from build123d import *

# Parameters (mm, degrees)
F1_DEPTH = 25.4
F3_R     = 39.2915838244
F4_DEPTH = 25.4
F6_R     = 62.7093604839
F7_DEPTH = 25.4
F8_T     = -2.54


with BuildPart() as f1:
    # F0 (on Front) → F1 (new body)
    with BuildSketch(Plane.XZ):
        with BuildLine():
            add(Edge.make_bspline(
                [(-55.208299309, 58.1508763134), (-67.0164708846, 55.3175541912), (-87.6445105915, -47.0922011076), (101.1268779134, 10.7779345683), (-19.4909088182, 79.2065756794), (-30.9714891326, 30.3974201797), (-47.8340446405, 59.9202983407), (-55.208299309, 58.1508763134)],
                knots=[0, 0, 0, 0, 0.2192278895, 0.4966401959, 0.7260839501, 0.8630912265, 1, 1, 1, 1], degree=3))
        make_face()
    extrude(amount=F1_DEPTH)


with BuildPart() as f4:
    # F3 (on Front) → F4 (new body)
    with BuildSketch(Plane.XZ):
        Circle(F3_R)
    extrude(amount=F4_DEPTH)


with BuildPart() as f7:
    # F6 (on Front) → F7 (new body)
    with BuildSketch(Plane.XZ):
        Circle(F6_R)
    extrude(amount=F7_DEPTH)

    # F8
    f8_openings = [f7.faces().sort_by_distance(p)[0] for p in [
        (0, -25.4, 0),
    ]]
    offset(amount=F8_T, openings=f8_openings)


solid = f7.part
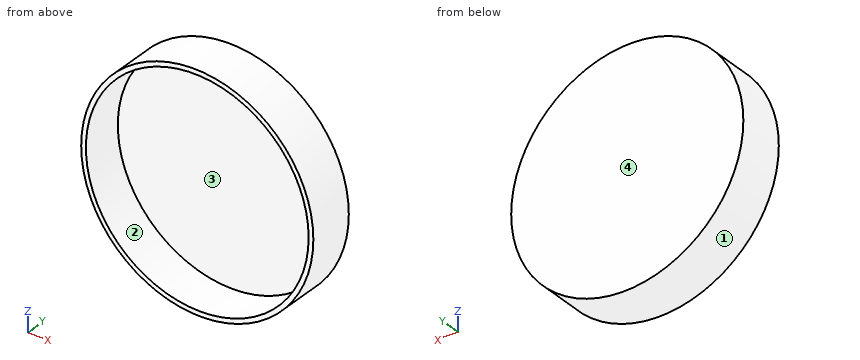
Can you work these out from the model? Positions are in its coordinate system, mm. Face numbers are marked on the shaded views. Coordinates: 2 decimals unless noted, no trailing zeros. Write each loop counter-clockwise with the first axis right and the second up, starting at its lowest first coordinate (ties: lowest second). Pieces come first, ordered by that corner, then holes. Notation, with made-up numbers: (60, -7) - (108, -7) arc R28 ccw to (108, 29) - close; hole circle Ø8 at (-35.5, -22.5). An arc over 180 degrees is marked (long way). Return JSON: item names as keys, results as strings. Group by question number.
Item 1: If we section it at B-B (z = 0): Write out the boundary of the cut face in (x, y), then the cut area to 3 significant figures.
Item 2: I'm going to push flat-ended pins straight in: pin 1 Ø10 at (x, y) = (16, -15) entering from -Z; pin 2 Ø3 at (x, z) = (-31.5, 16) entering from -Y; pin 3 Ø8 at (x, y) = (-25, -11) entering from -Z. Where does each tip first touch, or does it pass through?
Item 3: Please list where these lines run through material, in increasing order: probe 1 along Z at (x, y) = (0, -7.25); probe 2 along Y at (x, z) = (37.5, -36); probe 3 along X at (y, z) = (-19, 13.5).
Item 4: We'd pull the mould along Z, two halves only. Please class the marked faces 1, 2, 3 and 4: pulls with the +Z half, pulls with the -Z half, needs draft (parallel to the pull), parting line crosses it, or undercut.
Item 5: If we section it at C-C (y = -17.25): Write out the boundary of the cut face in (x, z).
Item 6: If we section it at A-A (x = 0): Write out the boundary of the cut face in (y, z).
Return value:
{
 "1": {"outline": "(-62.71, -25.4) - (-60.17, -25.4) - (-60.17, -2.54) - (60.17, -2.54) - (60.17, -25.4) - (62.71, -25.4) - (62.71, 0) - (-62.71, 0) - close", "area": "435 mm^2"},
 "2": {"pin 1": "stops at z = -61.74", "pin 2": "stops at y = -2.54", "pin 3": "stops at z = -59.09"},
 "3": {"probe 1": "z = -62.71 to -60.17, 60.17 to 62.71", "probe 2": "y = -2.54 to 0", "probe 3": "x = -61.24 to -58.64, 58.64 to 61.24"},
 "4": {"face 1": "parting line crosses it", "face 2": "undercut", "face 3": "undercut", "face 4": "needs draft"},
 "5": {"outline": "circle Ø125.42 at (0, 0); hole circle Ø120.34 at (0, 0)"},
 "6": {"outline": "(-25.4, -62.71) - (0, -62.71) - (0, 62.71) - (-25.4, 62.71) - (-25.4, 60.17) - (-2.54, 60.17) - (-2.54, -60.17) - (-25.4, -60.17) - close"}
}
